Work out the finished part from the listing and answer in its coordinate system (mm). Face numbers are marked on the shaded views. A direction names the side the tool comes from. Give positions to 0.01 mm unless a question says otherwise; leave off trailing zeros. Order: outer loops, then holes, each group sorted by start corner. A loop starts at its lowest first (then second) coordinate and runs counter-clockwise, first axis right, second up. Notation, with made-up numbers: (-13, 13.5) - (-9, 13.5) arc R4 cw to (-9, 20.5) - close; hole circle Ø5 at (66.5, 77.25). An arc over 180 degrees is marked (long way). Put each result on its own line as item: value.
```python
from build123d import *

# Parameters (mm, degrees)
F0_R     = 5
F0_R_2   = 2.5
F1_DEPTH = 3.5
F2_R     = 8
F2_R_2   = 2.5
F3_DEPTH = 1
F5_R     = 8
F5_R_2   = 2.5
F6_DEPTH = 7
F7_SIZE  = 1
F8_R     = 1.5
F9_DEPTH = 8.001


# Not quite as in the source:
# - a feature names something its author has since deleted; it is built from what else it names


with BuildPart() as f1:
    # F0 (on Top) → F1 (new body, symmetric)
    with BuildSketch(Plane.XY):
        Circle(F0_R)
        Circle(F0_R_2, mode=Mode.SUBTRACT)
    extrude(amount=F1_DEPTH, both=True)

    # F2 (on face) → F3 (join)
    with BuildSketch(Plane.XY.offset(3.5)):
        Circle(F2_R)
        Circle(F2_R_2, mode=Mode.SUBTRACT)
    extrude(amount=F3_DEPTH)

    # F4: F1 across plane


with BuildPart() as f1_1:
    add(f1.part)
    add(f1.part.mirror(Plane.XY))

    # F5 (on face) → F6 (join)
    with BuildSketch(Plane.XY.offset(4.5)):
        Circle(F5_R)
        Circle(F5_R_2, mode=Mode.SUBTRACT)
    extrude(amount=F6_DEPTH)

    # F7
    f7_edges = [f1_1.edges().sort_by_distance(p)[0] for p in [
        (-2.5, 0, 11.5),
        (-2.5, 0, -4.5),
    ]]
    chamfer(f7_edges, length=F7_SIZE)

    # F8 (on Front) → F9 (cut, through all)
    with BuildSketch(Plane.XZ):
        with Locations((0, 8)):
            Circle(F8_R)
    extrude(amount=-F9_DEPTH, mode=Mode.SUBTRACT)


solid = f1_1.part
```
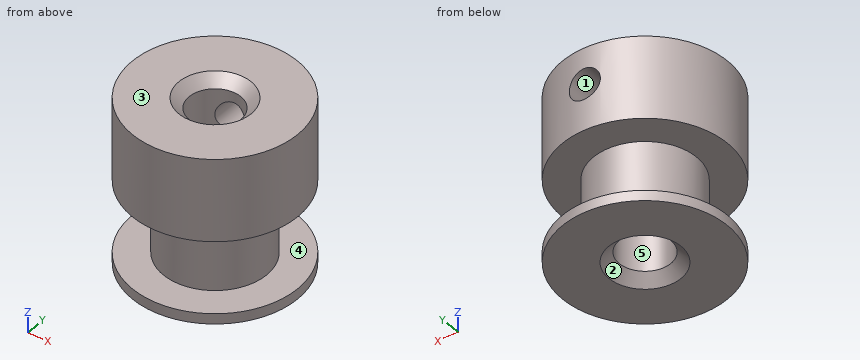
(1) Section C-C, the plane z = 5.5 is taken. Write down the section's boundary in (x, y).
Geometry check:
outline: circle Ø16 at (0, 0); hole circle Ø5 at (0, 0)
(2) A tool of negligible diameter and unlimited length cuts with its end or side. For the marked faces 4 and 5, from which of +Z, -Z, +X, -X, +Y, -Y can it reach the whole face along a straight path? Write none if from no direction.
Geometry check:
face 4: none
face 5: +Z, -Z
(3) Straight lines are drawn through the part: line 1 (Z direction, x = 3.5, y = 5.75); line 2 (Z direction, x = -0.75, y = 6.5); line 3 (Z direction, x = 0, y = 3.75). For each, find the intervals that lie inside material, in ascending order.
Geometry check:
line 1: z = -4.5 to -3.5, 3.5 to 11.5
line 2: z = -4.5 to -3.5, 3.5 to 6.7, 9.3 to 11.5
line 3: z = -4.5 to 6.5, 9.5 to 11.5
(4) Given pin 1 (4 mm diameter, centred on x = -2, y = 1.5, fed in from +Z); pin 2 (2.5 mm diameter, centred on x = 0, z = 8, fed in from +Y); pin 3 (1 mm diameter, centred on x = -4, z = 7.5, fed in from +Y); pin 4 (2 mm diameter, centred on x = 1, y = 1.5, fed in from +Z), each flat-ended and moving along its own axis, determine where each tip first touches the part or whether it passes through.
Geometry check:
pin 1: stops at z = 11.5
pin 2: stops at y = -2.17
pin 3: stops at y = 7.19
pin 4: stops at z = 10.8
(5) Determine the mould class of the marked faces 1, 2 and 3 for opening direction Z: pulls with the +Z half, pulls with the -Z half, needs draft (parallel to the pull), parting line crosses it, or undercut.
Geometry check:
face 1: undercut
face 2: pulls with the -Z half
face 3: pulls with the +Z half
(6) Section B-B, the plane x = 0 is taken. Write down the section's boundary in (y, z).
Geometry check:
outline: (-8, -4.5) - (-3.5, -4.5) - (-2.5, -3.5) - (-2.5, 10.5) - (-3.5, 11.5) - (-8, 11.5) - (-8, 3.5) - (-5, 3.5) - (-5, -3.5) - (-8, -3.5) - close; (2.5, -3.5) - (3.5, -4.5) - (8, -4.5) - (8, -3.5) - (5, -3.5) - (5, 3.5) - (8, 3.5) - (8, 6.5) - (2.5, 6.5) - close; (2.5, 9.5) - (8, 9.5) - (8, 11.5) - (3.5, 11.5) - (2.5, 10.5) - close
(7) Section D-D, the plane y = -4.5 is taken. Write down the section's boundary in (x, z).
Geometry check:
outline: (-6.61, -4.5) - (6.61, -4.5) - (6.61, -3.5) - (2.18, -3.5) - (2.18, 3.5) - (6.61, 3.5) - (6.61, 11.5) - (-6.61, 11.5) - (-6.61, 3.5) - (-2.18, 3.5) - (-2.18, -3.5) - (-6.61, -3.5) - close
(8) Section A-A, the plane y = 0 is taken. Write down the section's boundary in (x, z).
Geometry check:
outline: (-8, -4.5) - (-3.5, -4.5) - (-2.5, -3.5) - (-2.5, 10.5) - (-3.5, 11.5) - (-8, 11.5) - (-8, 3.5) - (-5, 3.5) - (-5, -3.5) - (-8, -3.5) - close; (2.5, -3.5) - (3.5, -4.5) - (8, -4.5) - (8, -3.5) - (5, -3.5) - (5, 3.5) - (8, 3.5) - (8, 11.5) - (3.5, 11.5) - (2.5, 10.5) - close
